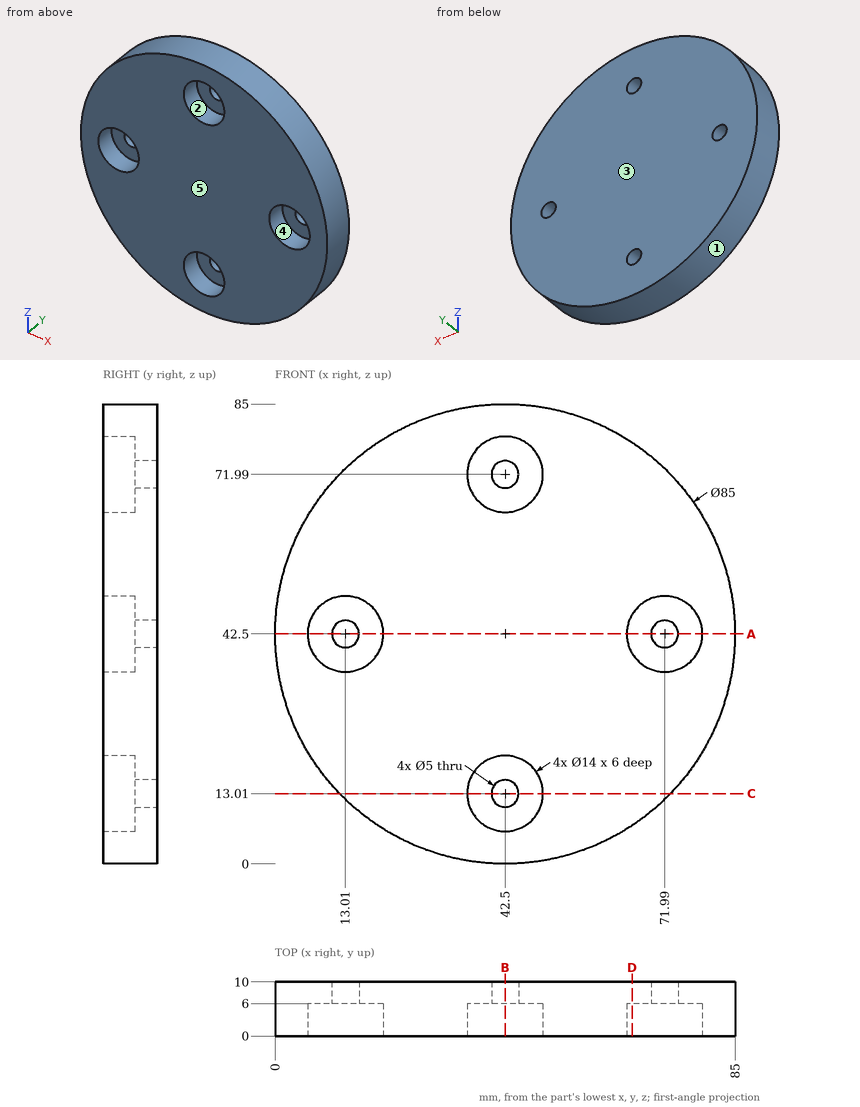
Job drawing, mm, ordinate dimensions from the low corner. One solid piece. A direction names the side the tool comes from. Coordinates: 2 decimals unless noted, no trailing zeros. Order: outer loops, then holes, each group sorted by start corner. A loop starts at its lowest first (then second) coordinate and runs counter-clockwise, first axis right, second up. Notation, with made-up numbers: (85, 1.5) -> (123, 1.5) arc R16 ccw to (123, 18.5) -> close; hole circle Ø2 at (1.25, 54). An arc over 180 degrees is marked (long way). Return JSON: item names as keys, results as strings. Group by question number.
Item 1: Saw through at D-D on x = 66. Write the cut outline in (y, z), then the cut area to 3 significant figures.
Item 2: Saw through at A-A on z = 42.5. Write the cut outline in (x, y).
Item 3: Saw through at C-C on z = 13. Write the cut outline in (x, y).
Item 4: Saw through at B-B on x = 42.5. Write the cut outline in (y, z), then the cut area to 3 significant figures.
Item 5: Pull direction Z, two halves, no side cores. Call the marked faces 1, 2 and 3: pulls with the +Z half, pulls with the -Z half, needs draft (parallel to the pull), parting line crosses it, or undercut.
Item 6: Wall check: line 1 along X through (y, z) = (5.25, 43); line 2 along X through (y, z) = (5, 74) (1 decimal); line 3 along X through (y, z) = (3, 66.5) (1 decimal). Give the ranges that are in metal, low to high. Write a range as [from, to].
Item 7: Tool access for the marked faces 4 and 5: list every direction of +Z, -Z, +X, -X, +Y, -Y with a clear straight run to the whole face (end or side of a thin tool).
Item 8: Flat gauge pins, fed straight in: P1, Ø18, axis at x = 42.5, z = 71.99, coming from the +Y side; P2, Ø2, axis at y = 3, z = 14.5, coming from the -X side; P3, Ø7, axis at x = 42.5, z = 71, coming from the -Y side; P4, Ø3, axis at y = 3.5, z = 55, coming from the -X side. Where does each tip first touch, or does it go through?
Values found:
{
 "1": {"outline": "(0, 7.09) -> (10, 7.09) -> (10, 77.91) -> (0, 77.91) -> (0, 46.12) -> (6, 46.12) -> (6, 38.88) -> (0, 38.88) -> close", "area": "665 mm2"},
 "2": {"outline": "(0, 0) -> (6.01, 0) -> (6.01, 6) -> (10.51, 6) -> (10.51, 10) -> (0, 10) -> close; (15.51, 6) -> (20.01, 6) -> (20.01, 0) -> (64.99, 0) -> (64.99, 6) -> (69.49, 6) -> (69.49, 10) -> (15.51, 10) -> close; (74.49, 6) -> (78.99, 6) -> (78.99, 0) -> (85, 0) -> (85, 10) -> (74.49, 10) -> close"},
 "3": {"outline": "(11.91, 0) -> (35.5, 0) -> (35.5, 6) -> (40, 6) -> (40, 10) -> (11.91, 10) -> close; (45, 6) -> (49.5, 6) -> (49.5, 0) -> (73.09, 0) -> (73.09, 10) -> (45, 10) -> close"},
 "4": {"outline": "(0, 0) -> (10, 0) -> (10, 10.51) -> (6, 10.51) -> (6, 6.01) -> (0, 6.01) -> close; (0, 20.01) -> (6, 20.01) -> (6, 15.51) -> (10, 15.51) -> (10, 69.49) -> (6, 69.49) -> (6, 64.99) -> (0, 64.99) -> close; (0, 78.99) -> (6, 78.99) -> (6, 74.49) -> (10, 74.49) -> (10, 85) -> (0, 85) -> close", "area": "642 mm2"},
 "5": {"face 1": "parting line crosses it", "face 2": "undercut", "face 3": "needs draft"},
 "6": {"line 1": "x = [0, 6.03], [19.99, 65.01], [78.97, 85]", "line 2": "x = [14, 35.8], [49.2, 71]", "line 3": "x = [7.4, 38.2], [46.8, 77.6]"},
 "7": {"face 4": "-Y", "face 5": "+Z, -Z, +X, -X, -Y"},
 "8": {"P1": "stops at y = 10", "P2": "stops at x = 9.68", "P3": "stops at y = 6", "P4": "stops at x = 1.45"}
}
